The listing builds one solid part. Answer for the finished solid, in the listing's coordinates (mm). A direction names the side the tool comes from. Give positions to 0.01 mm unless a question says otherwise; leave off trailing zeros. Write each loop counter-clockwise with the first axis right and the second up, starting at its lowest first coordinate (ties: lowest second). Pieces come first, ordered by that corner, then holes. Notation, with made-up numbers: M -38,-2 L -28,-2 A13 ccw -28,14 Z; hole C 88,60.5 d10. An arc over 180 degrees is marked long. Answer as a JSON object with one key per item and string values.
```python
from build123d import *

# Parameters (mm, degrees)
SKETCH2_W             = 53.8
SKETCH2_H             = 39.8
BOSS_EXTRUDE1_DEPTH   = 12
SKETCH3_W             = 70
SKETCH3_H             = 60
BOSS_EXTRUDE2_DEPTH   = 31.5
SKETCH4_R             = 2.1
CUT_EXTRUDE1_DEPTH    = 50.9
SKETCH5_W             = 36
SKETCH5_H             = 39.8
CUT_EXTRUDE2_DEPTH    = 12
CHAMFER1_SIZE         = 0.5
CHAMFER1_SIZE2        = 1.37373871
CHAMFER1_PART_2_SIZE  = 0.5
CHAMFER1_PART_2_SIZE2 = 1.37373871
CUT_EXTRUDE13_DEPTH   = 61


with BuildPart() as part:
    # Sketch2 → Boss-Extrude1 (new body)
    with BuildSketch(Plane.XY):
        Rectangle(SKETCH2_W, SKETCH2_H)
    extrude(amount=BOSS_EXTRUDE1_DEPTH)

    # Sketch3 → Boss-Extrude2 (add)
    with BuildSketch(Plane.XY.offset(12)):
        Rectangle(SKETCH3_W, SKETCH3_H)
    extrude(amount=BOSS_EXTRUDE2_DEPTH)

    # Sketch4 → Cut-Extrude1 (cut, through all)
    with BuildSketch(Plane(origin=(0, 19.9, 0), x_dir=(1, 0, 0), z_dir=(0, 1, 0))):
        with Locations((22.5, -4.6)):
            Circle(SKETCH4_R)
        with Locations((-22.5, -4.6)):
            Circle(SKETCH4_R)
    extrude(amount=-CUT_EXTRUDE1_DEPTH, mode=Mode.SUBTRACT)

    # Sketch5 → Cut-Extrude2 (cut)
    with BuildSketch(Plane(origin=(0, 0, 0), x_dir=(-1, 0, 0), z_dir=(0, 0, -1))):
        Rectangle(SKETCH5_W, SKETCH5_H)
    extrude(amount=-CUT_EXTRUDE2_DEPTH, mode=Mode.SUBTRACT)

    # Chamfer1
    chamfer1_edges = [part.edges().sort_by_distance(p)[0] for p in [
        (-22.45, 19.9, 0),
        (-18, 0, 0),
        (-22.45, -19.9, 0),
        (-26.9, 0, 0),
    ]]
    chamfer1_side = [part.faces().sort_by_distance(p)[0] for p in [
        (-22.45, 0, 0),
    ]]
    chamfer(chamfer1_edges, length=CHAMFER1_SIZE, length2=CHAMFER1_SIZE2, reference=chamfer1_side[0])

    # Chamfer1 part 2
    chamfer1_part_2_edges = [part.edges().sort_by_distance(p)[0] for p in [
        (22.45, -19.9, 0),
        (18, 0, 0),
        (22.45, 19.9, 0),
        (26.9, 0, 0),
    ]]
    chamfer1_part_2_side = [part.faces().sort_by_distance(p)[0] for p in [
        (22.45, 0, 0),
    ]]
    chamfer(chamfer1_part_2_edges, length=CHAMFER1_PART_2_SIZE, length2=CHAMFER1_PART_2_SIZE2, reference=chamfer1_part_2_side[0])

    # Sketch27 → Cut-Extrude13 (cut, through all)
    with BuildSketch(Plane.XZ.offset(30)):
        with BuildLine():
            ThreePointArc((-35, 14), (0, 25.266028276), (35, 14))
            ThreePointArc((35, 14), (0, 140.049707845), (-35, 14))
        make_face()
    extrude(amount=-CUT_EXTRUDE13_DEPTH, mode=Mode.SUBTRACT)


solid = part.part
```
1. A cutting plane is placed at B-B, the plane z = 4.6. Give the vertices of the cut face in (x, y), plus the area to 3 significant figures.
Verdict:
{"outline": "M -26.9,-19.9 L -24.6,-19.9 L -24.6,19.9 L -26.9,19.9 Z; M -20.4,-19.9 L -18,-19.9 L -18,19.9 L -20.4,19.9 Z; M 18,-19.9 L 20.4,-19.9 L 20.4,19.9 L 18,19.9 Z; M 24.6,-19.9 L 26.9,-19.9 L 26.9,19.9 L 24.6,19.9 Z", "area": "374 mm2"}
2. Consider line 1 along X through (y, z) = (-1, 4.6); line 2 along X through (y, z) = (-13, 8); line 3 along Y through (x, z) = (-25, 1.75). Determine where each line is inside the solid, lowest interval first.
Verdict:
{"line 1": "x = -26.9 to -24.6, -20.4 to -18, 18 to 20.4, 24.6 to 26.9", "line 2": "x = -26.9 to -18, 18 to 26.9", "line 3": "y = -19.9 to 19.9"}
3. The mould has two halves that part along Z. Classify faces 1 (the flat face through (-23, 0, 0)), 2 (the cylindrical face through (23.469, 0.279, 6.463)), 3 (the flat face through (-18, 0, 7)), 4 (the cylindrical face through (-21.531, 0.279, 6.463)): released by +Z, released by -Z, zero draft, split by the parting line, or undercut.
Verdict:
{"face 1": "released by -Z", "face 2": "undercut", "face 3": "zero draft", "face 4": "undercut"}
4. A cutting plane is placed at A-A, the plane z = 8.25. Give the vertices of the cut face in (x, y).
Verdict:
{"outline": "M -26.9,-19.9 L -18,-19.9 L -18,19.9 L -26.9,19.9 Z; M 18,-19.9 L 26.9,-19.9 L 26.9,19.9 L 18,19.9 Z"}
5. For faces 5 (the flat face through (-23, 19.9, 8)), 6 (the flat face through (18, 0, 7)), 7 (the flat face through (26.9, 0, 7)), 8 (the flat face through (-26.9, 0, 7)), determine the directions among +Z, -Z, +X, -X, +Y, -Y from which every point of the face is accessible in a straight line to the end or side of a thin tool.
Verdict:
{"face 5": "-Z, +X, -X, +Y", "face 6": "-Z, +Y, -Y", "face 7": "-Z, +X, +Y, -Y", "face 8": "-Z, -X, +Y, -Y"}
6. A cutting plane is placed at D-D, the plane x = 22.5. Give the vertices of the cut face in (y, z), plus the area to 3 significant figures.
Verdict:
{"outline": "M -30,12 L -19.9,12 L -19.9,6.7 L 19.9,6.7 L 19.9,12 L 30,12 L 30,20.89 L -30,20.89 Z; M -19.9,1.37 L -19.4,0 L 19.4,0 L 19.9,1.37 L 19.9,2.5 L -19.9,2.5 Z", "area": "843 mm2"}
7. Flat-ended cylindrical pins translate along their axes: pin 1 (6.5 mm diameter, centred on x = -22.5, z = 4.6, fed in from -Y); pin 2 (5.5 mm diameter, centred on y = 1.5, z = 4, fed in from +X); pin 3 (1 mm diameter, centred on x = 1, y = 17.5, fed in from -Z); pin 4 (18 mm diameter, centred on x = -12.5, y = -14, fed in from -Z). Find the tip coordinate at first contact, or state that the pin passes through.
Verdict:
{"pin 1": "stops at y = -19.9", "pin 2": "stops at x = 26.9", "pin 3": "stops at z = 12", "pin 4": "stops at z = 0"}
8. A cutting plane is placed at C-C, the plane y = 15. Give the vertices of the cut face in (x, z).
Verdict:
{"outline": "M -35,12 L -26.9,12 L -26.9,1.37 L -26.4,0 L -18.5,0 L -18,1.37 L -18,12 L 18,12 L 18,1.37 L 18.5,0 L 26.4,0 L 26.9,1.37 L 26.9,12 L 35,12 L 35,14 A60 ccw -35,14 Z; hole C -22.5,4.6 d4.2; hole C 22.5,4.6 d4.2"}
